For this review, take the finished solid that the model builds, in its own axes (mm). Coordinates: 2 decimals unless noted, no trailing zeros. Loops run counter-clockwise (first coordinate to the right, second up) from the corner with the lowest first, then second, coordinate; pieces in that order, holes last. Notation, with made-up numbers: (-9, -25.5) -> (15, -25.5) arc R22 ccw to (15, -16.5) -> close; hole circle Ø7 at (20, 14). An arc over 180 degrees is marked (long way). Use a Markdown table: item, result.
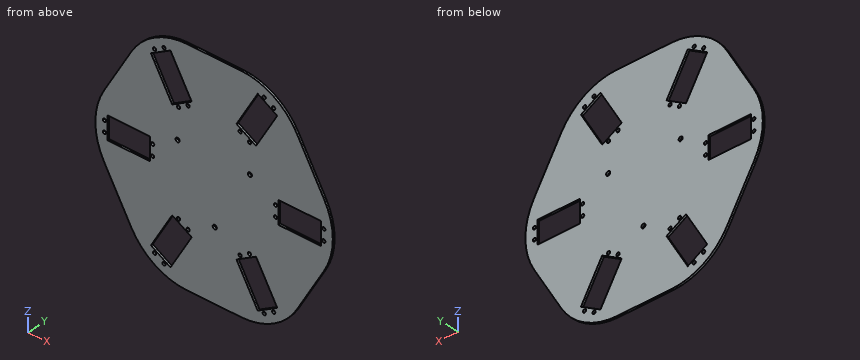
from build123d import *

# Parameters (mm, degrees)
SKETCH1_R           = 2.5
SKETCH1_W           = 66
SKETCH1_H           = 35
BOSS_EXTRUDE1_DEPTH = 3.175
SKETCH2_R           = 3.2
CUT_EXTRUDE1_DEPTH  = 3.175


with BuildPart() as part:
    # Sketch1 → Boss-Extrude1 (new body)
    with BuildSketch(Plane(origin=(0, 0, 0), x_dir=(1, 0, 0), z_dir=(0, 1, 0))):
        with BuildLine():
            Line((171.132486541, 50), (128.867513459, 123.205080757))
            ThreePointArc((128.867513459, 123.205080757), (92.264973081, 159.807621135), (42.264973081, 173.205080757))
            Line((42.264973081, 173.205080757), (-42.264973081, 173.205080757))
            ThreePointArc((-42.264973081, 173.205080757), (-92.264973081, 159.807621135), (-128.867513459, 123.205080757))
            Line((-128.867513459, 123.205080757), (-171.132486541, 50))
            ThreePointArc((-171.132486541, 50), (-184.529946162, 0), (-171.132486541, -50))
            Line((-171.132486541, -50), (-128.867513459, -123.205080757))
            ThreePointArc((-128.867513459, -123.205080757), (-92.264973081, -159.807621135), (-42.264973081, -173.205080757))
            Line((-42.264973081, -173.205080757), (42.264973081, -173.205080757))
            ThreePointArc((42.264973081, -173.205080757), (92.264973081, -159.807621135), (128.867513459, -123.205080757))
            Line((128.867513459, -123.205080757), (171.132486541, -50))
            ThreePointArc((171.132486541, -50), (184.529946162, 0), (171.132486541, 50))
        make_face()
        with Locations(Location((170.5, 8.5, 0), (0, 0, 270))):
            Circle(SKETCH1_R, mode=Mode.SUBTRACT)
        with Locations(Location((170.5, -8.5, 0), (0, 0, 270))):
            Circle(SKETCH1_R, mode=Mode.SUBTRACT)
        with Locations(Location((95.5, 8.5, 0), (0, 0, 270))):
            Circle(SKETCH1_R, mode=Mode.SUBTRACT)
        with Locations(Location((95.5, -8.5, 0), (0, 0, 270))):
            Circle(SKETCH1_R, mode=Mode.SUBTRACT)
        with Locations(Location((40.388784068, -86.955426061, 0), (0, 0, 270))):
            Circle(SKETCH1_R, mode=Mode.SUBTRACT)
        with Locations(Location((55.111215932, -78.455426061, 0), (0, 0, 270))):
            Circle(SKETCH1_R, mode=Mode.SUBTRACT)
        with Locations(Location((92.611215932, -143.407331345, 0), (0, 0, 270))):
            Circle(SKETCH1_R, mode=Mode.SUBTRACT)
        with Locations(Location((77.888784068, -151.907331345, 0), (0, 0, 270))):
            Circle(SKETCH1_R, mode=Mode.SUBTRACT)
        with Locations(Location((-55.111215932, -78.455426061, 0), (0, 0, 270))):
            Circle(SKETCH1_R, mode=Mode.SUBTRACT)
        with Locations(Location((-40.388784068, -86.955426061, 0), (0, 0, 270))):
            Circle(SKETCH1_R, mode=Mode.SUBTRACT)
        with Locations(Location((-77.888784068, -151.907331345, 0), (0, 0, 270))):
            Circle(SKETCH1_R, mode=Mode.SUBTRACT)
        with Locations(Location((-92.611215932, -143.407331345, 0), (0, 0, 270))):
            Circle(SKETCH1_R, mode=Mode.SUBTRACT)
        with Locations(Location((-95.5, 8.5, 0), (0, 0, 270))):
            Circle(SKETCH1_R, mode=Mode.SUBTRACT)
        with Locations(Location((-95.5, -8.5, 0), (0, 0, 270))):
            Circle(SKETCH1_R, mode=Mode.SUBTRACT)
        with Locations(Location((-170.5, -8.5, 0), (0, 0, 270))):
            Circle(SKETCH1_R, mode=Mode.SUBTRACT)
        with Locations(Location((-170.5, 8.5, 0), (0, 0, 270))):
            Circle(SKETCH1_R, mode=Mode.SUBTRACT)
        with Locations(Location((-40.388784068, 86.955426061, 0), (0, 0, 270))):
            Circle(SKETCH1_R, mode=Mode.SUBTRACT)
        with Locations(Location((-55.111215932, 78.455426061, 0), (0, 0, 270))):
            Circle(SKETCH1_R, mode=Mode.SUBTRACT)
        with Locations(Location((-92.611215932, 143.407331345, 0), (0, 0, 270))):
            Circle(SKETCH1_R, mode=Mode.SUBTRACT)
        with Locations(Location((-77.888784068, 151.907331345, 0), (0, 0, 270))):
            Circle(SKETCH1_R, mode=Mode.SUBTRACT)
        with Locations(Location((55.111215932, 78.455426061, 0), (0, 0, 270))):
            Circle(SKETCH1_R, mode=Mode.SUBTRACT)
        with Locations(Location((40.388784068, 86.955426061, 0), (0, 0, 270))):
            Circle(SKETCH1_R, mode=Mode.SUBTRACT)
        with Locations(Location((77.888784068, 151.907331345, 0), (0, 0, 270))):
            Circle(SKETCH1_R, mode=Mode.SUBTRACT)
        with Locations(Location((92.611215932, 143.407331345, 0), (0, 0, 270))):
            Circle(SKETCH1_R, mode=Mode.SUBTRACT)
        with Locations((133, 0)):
            Rectangle(SKETCH1_W, SKETCH1_H, mode=Mode.SUBTRACT)
        Polygon((65.155444566, -77.852540378), (98.155444566, -135.010217028), (67.844555434, -152.510217028), (34.844555434, -95.352540378), align=None, mode=Mode.SUBTRACT)
        Polygon((-34.844555434, -95.352540378), (-67.844555434, -152.510217028), (-98.155444566, -135.010217028), (-65.155444566, -77.852540378), align=None, mode=Mode.SUBTRACT)
        with Locations((-133, 0)):
            Rectangle(SKETCH1_W, SKETCH1_H, mode=Mode.SUBTRACT)
        Polygon((-65.155444566, 77.852540378), (-98.155444566, 135.010217028), (-67.844555434, 152.510217028), (-34.844555434, 95.352540378), align=None, mode=Mode.SUBTRACT)
        Polygon((34.844555434, 95.352540378), (67.844555434, 152.510217028), (98.155444566, 135.010217028), (65.155444566, 77.852540378), align=None, mode=Mode.SUBTRACT)
    extrude(amount=BOSS_EXTRUDE1_DEPTH)

    # Sketch2 → Cut-Extrude1 (cut)
    with BuildSketch(Plane(origin=(0, 3.175, 0), x_dir=(1, 0, 0), z_dir=(0, 1, 0))):
        with Locations(Location((55.794244464, -33.346698257, 0), (0, 0, 270))):
            Circle(SKETCH2_R)
        with Locations(Location((-56.776210055, -31.645883963, 0), (0, 0, 270))):
            Circle(SKETCH2_R)
        with Locations(Location((0.981965591, 64.99258222, 0), (0, 0, 270))):
            Circle(SKETCH2_R)
    extrude(amount=-CUT_EXTRUDE1_DEPTH, mode=Mode.SUBTRACT)


solid = part.part
(1) For line 1 along Z through (x, y) = (57, 2.85); line 2 along Z through (x, y) = (-65, 1.95); line 3 along X through (y, z) = (2, 138.5), list the stretches that pass through material, from the lowest coordinate up.
Found:
| item | result |
|---|---|
| line 1 | z = -172.11 to -133.73, -82.56 to -80.09, -76.82 to 30.38, 36.31 to 76.82, 80.09 to 82.56, 133.73 to 172.11 |
| line 2 | z = -170.59 to -147.58, -77.94 to 77.94, 147.58 to 170.59 |
| line 3 | x = -118.01 to -92.11, -59.76 to 59.76, 92.11 to 118.01 |
(2) Take a section at A-A on x = -116. Write out the cut boundary in (y, z) (3 decimals), plus the area to 3 significant figures.
Found:
| item | result |
|---|---|
| outline | (0, -140.756) -> (3.175, -140.756) -> (3.175, -17.5) -> (0, -17.5) -> close; (0, 17.5) -> (3.175, 17.5) -> (3.175, 140.756) -> (0, 140.756) -> close |
| area | 783 mm^2 |
(3) Take a section at B-B on y = 1.4. State how many separate pieces and enclosed holes the cut face has, plus the area to 3 significant figures.
Found:
| item | result |
|---|---|
| separate pieces | 1 |
| enclosed holes | 33 |
| area | 86,300 mm^2 |
(4) For pin 1 Ø3 at (x, z) = (-92.61, -143.41) entering from +Y; pin 2 Ø1.6 at (x, y) = (140, 2) entering from -Z; pin 3 Ø1 at (y, z) = (2, -8) entering from -X; pin 4 Ø1.5 at (x, y) = (112, 1) entering from -Z, all flat-tipped, find the tip position at first contact; note any pin that passes through.
Found:
| item | result |
|---|---|
| pin 1 | passes through |
| pin 2 | stops at z = -105.31 |
| pin 3 | stops at x = -184.25 |
| pin 4 | stops at z = -145.6 |
(5) Take a section at C-C on x = -153. Write out the cut boundary in (y, z) (3 decimals), plus the area to 3 significant figures.
Found:
| item | result |
|---|---|
| outline | (0, -81.406) -> (3.175, -81.406) -> (3.175, -17.5) -> (0, -17.5) -> close; (0, 17.5) -> (3.175, 17.5) -> (3.175, 81.406) -> (0, 81.406) -> close |
| area | 406 mm^2 |
